Autodesk Inventor part; units mm, degrees
ref_plane "YZ Plane" through (0, 0, 0) normal (1, 0, 0) x (0, 1, 0)
ref_plane "XZ Plane" through (0, 0, 0) normal (0, 1, 0) x (-1, 0, 0)
ref_plane "XY Plane" through (0, 0, 0) normal (0, 0, 1) x (1, 0, 0)
ref_plane "Work Plane1" through (0, 0, 0) normal (0, 0, 1) x (1, 0, 0)
sketch "Sketch1" plane through (0, 0, 0) normal (0, 0, 1) x (1, 0, 0)
  circle A0 centre (0, 0) radius 25.9979
  circle A1 centre (-9.4998, -11.0022) radius 2.6601
  circle A2 centre (0.0001, -0.0022) radius 3.8801
  circle A3 centre (0.0001, -0.0022) radius 6.7754
  point P0 (0, 0)
extrude "Extrusion1" add sketch "Sketch1" along normal blind 7 contours A0
sketch "Sketch2" plane through (0, 0, 7) normal (0, 0, 1) x (1, 0, 0)
  line L0 (-10.4551, 50.2837) -> (48.898, -9.0695)
  line L1 (48.898, -9.0695) -> (20.6137, -37.3537)
  line L2 (20.6137, -37.3537) -> (-38.7394, 21.9994)
  line L3 (-38.7394, 21.9994) -> (-10.4551, 50.2837)
  line L4 (-10.4551, 50.2837) -> (20.6137, -37.3537) construction
  line L5 (48.898, -9.0695) -> (-38.7394, 21.9994) construction
  line L6 (-10.4551, 50.2837) -> (73.4829, 50.2837) construction
  circle A0 centre (-9.4998, -11.0022) radius 2.6601
  point P0 (5.0793, 6.465)
  dimension "d2" = 135
  dimension "d3" = 40
extrude "Extrusion2" cut sketch "Sketch2" against normal blind 2.5 contours L0 L1 L2 L3
sketch "Sketch3" plane through (0, 0, 7) normal (0, 0, 1) x (1, 0, 0)
  line L0 (-7.7936, -20.2561) -> (-2.9652, -15.4277)
  line L1 (-18.7537, -9.2959) -> (-13.9253, -4.4675)
  line L2 (-13.219, -3.6198) -> (-2.1175, -14.7214)
  line L3 (-2.1175, -14.7214) -> (-8.2078, -20.8117)
  line L4 (-8.2078, -20.8117) -> (-19.3094, -9.7102)
  line L5 (-19.3094, -9.7102) -> (-13.219, -3.6198)
  line L6 (-7.6188, -9.1212) -> (-24.7373, 7.9973)
  line L7 (-13.1696, -3.5704) -> (-2.1175, -14.7214)
  line L8 (-2.1175, -14.7214) -> (-0.0463, -12.6686)
  line L9 (-0.0463, -12.6686) -> (-11.0984, -1.5176)
  line L10 (-11.0984, -1.5176) -> (-13.1696, -3.5704)
  line L11 (-13.1696, -3.5704) -> (-13.219, -3.6198)
  line L12 (7.9973, -24.7373) -> (-24.7373, 7.9973)
  line L13 (-13.9253, -4.4675) -> (-2.9652, -15.4277)
  line L14 (-7.7936, -20.2561) -> (-18.7537, -9.2959)
  point P0 (0, 0)
  point P1 (-8.9176, -8.4066)
  point P2 (-24.7373, 7.9973)
  dimension "d6" = 0.1
extrude "Extrusion3" cut sketch "Sketch3" against normal up to surface (2.5 mm away) contours L14 L1 L13 L0 | L11 L7 L2 | L2 L3 L4 L5 | L7 L6 L12 L8 | L10 L9 L8 L12 L6
sketch "Skizze4" plane through (0, 0, 7) normal (0, 0, 1) x (1, 0, 0)
  spline S0 degree 2 poles (24.1427, 2.2394) (24.731, 1.8489) (25.3785, 0.5587) (25.3785, -0.3311) knots 0 0 0 1 2 2 2 construction
  spline S1 degree 2 poles (25.3785, -0.3311) (25.3785, -1.1665) (24.7013, -2.5111) (24.1328, -2.8867) knots 0 0 0 1 2 2 2 construction
  spline S2 degree 2 poles (24.1328, -2.8867) (23.6682, -3.1784) (22.7141, -3.3761) (21.9726, -3.3761) knots 0 0 0 1 2 2 2 construction
  line L0 (21.9726, -3.3761) -> (20.5687, -3.3761) construction
  line L1 (20.5687, -3.3761) -> (20.5687, 2.7239) construction
  line L2 (20.5687, 2.7239) -> (21.9578, 2.7239) construction
  spline S3 degree 2 poles (21.9578, 2.7239) (22.8179, 2.7239) (23.7967, 2.4668) (24.1427, 2.2394) knots 0 0 0 1 2 2 2 construction
  spline S4 degree 2 poles (19.1896, -2.9312) (18.8979, -3.1982) (18.1564, -3.4849) (17.5978, -3.4849) knots 0 0 0 1 2 2 2 construction
  spline S5 degree 2 poles (17.5978, -3.4849) (16.9354, -3.4849) (16.0061, -3.2081) (15.5958, -3.0103) knots 0 0 0 1 2 2 2 construction
  line L3 (15.5958, -3.0103) -> (15.5958, -1.992) construction
  line L4 (15.5958, -1.992) -> (15.6551, -1.992) construction
  spline S6 degree 2 poles (15.6551, -1.992) (16.0555, -2.3677) (17.0689, -2.7829) (17.5385, -2.7829) knots 0 0 0 1 2 2 2 construction
  spline S7 degree 2 poles (17.5385, -2.7829) (18.2108, -2.7829) (18.8979, -2.2243) (18.8979, -1.7646) knots 0 0 0 1 2 2 2 construction
  spline S8 degree 2 poles (18.8979, -1.7646) (18.8979, -1.3988) (18.5371, -0.944) (18.1465, -0.8303) knots 0 0 0 1 2 2 2 construction
  spline S9 degree 2 poles (18.1465, -0.8303) (17.8648, -0.7513) (17.3952, -0.6425) (17.0442, -0.5535) knots 0 0 0 1 2 2 2 construction
  spline S10 degree 2 poles (17.0442, -0.5535) (16.7278, -0.4695) (16.2285, -0.2174) (16.0358, -0.0147) knots 0 0 0 1 2 2 2 construction
  spline S11 degree 2 poles (16.0358, -0.0147) (15.8479, 0.188) (15.6403, 0.7317) (15.6403, 1.0876) knots 0 0 0 1 2 2 2 construction
  spline S12 degree 2 poles (15.6403, 1.0876) (15.6403, 1.8291) (16.797, 2.8326) (17.6918, 2.8326) knots 0 0 0 1 2 2 2 construction
  spline S13 degree 2 poles (17.6918, 2.8326) (18.2059, 2.8326) (19.1154, 2.6299) (19.5059, 2.4372) knots 0 0 0 1 2 2 2 construction
  line L5 (19.5059, 2.4372) -> (19.5059, 1.4683) construction
  line L6 (19.5059, 1.4683) -> (19.4466, 1.4683) construction
  spline S14 degree 2 poles (19.4466, 1.4683) (19.155, 1.7352) (18.2454, 2.1307) (17.7461, 2.1307) knots 0 0 0 1 2 2 2 construction
  spline S15 degree 2 poles (17.7461, 2.1307) (17.1826, 2.1307) (16.4856, 1.6017) (16.4856, 1.1717) knots 0 0 0 1 2 2 2 construction
  spline S16 degree 2 poles (16.4856, 1.1717) (16.4856, 0.7861) (16.8959, 0.3264) (17.2815, 0.2226) knots 0 0 0 1 2 2 2 construction
  spline S17 degree 2 poles (17.2815, 0.2226) (17.5385, 0.1534) (18.285, -0.0246) (18.5321, -0.0987) knots 0 0 0 1 2 2 2 construction
  spline S18 degree 2 poles (18.5321, -0.0987) (19.1599, -0.2915) (19.7432, -1.0676) (19.7432, -1.6361) knots 0 0 0 1 2 2 2 construction
  spline S19 degree 2 poles (19.7432, -1.6361) (19.7432, -1.997) (19.4516, -2.689) (19.1896, -2.9312) knots 0 0 0 1 2 2 2 construction
  circle A0 centre (-9.9998, 17.4978) radius 1.3999 construction
  circle A1 centre (10.0001, 17.4979) radius 1.4 construction
  circle A2 centre (10.0001, -17.5021) radius 1.4 construction
  circle A3 centre (-9.9998, -17.5021) radius 1.4001 construction
  arc A4 (-25.1198, 6.6998) -> (-24.1417, 5.4917) centre (-24.1417, 6.4917) ccw construction
  line L7 (-24.1417, 5.4917) -> (-17.7002, 5.4917) construction
  arc A5 (-15.7002, 3.4917) -> (-17.7002, 5.4917) centre (-17.7002, 3.4917) ccw construction
  line L8 (-15.7002, 3.4917) -> (-15.7002, -4.496) construction
  arc A6 (-17.7002, -6.496) -> (-15.7002, -4.496) centre (-17.7002, -4.496) ccw construction
  line L9 (-17.7002, -6.496) -> (-23.8502, -6.496) construction
  arc A7 (-23.8502, -6.496) -> (-24.8235, -7.7254) centre (-23.8502, -7.496) ccw construction
  arc A8 (-24.8235, -7.7254) -> (-25.1198, 6.6998) centre (0, 0) ccw construction
  circle A9 centre (-9.4998, -11.0022) radius 2.6601 construction
  circle A10 centre (-16.8291, -16.0482) radius 1.4 construction
  circle A11 centre (6.1284, 23.0202) radius 1.4 construction
  circle A12 centre (22.7119, 7.1872) radius 1.4 construction
  circle A13 centre (0.0001, -0.0022) radius 6.5 construction
  point P0 (0, 0)
hole "Bohrung1" at (6.1284, 23.0202, 7) at (22.7119, 7.1872, 7) at (-16.8291, -16.0482, 7) direction (0, 0, -1) diameter 3.2 end through all counterbore diameter 6.5 counterbore depth 5.5
sketch "Skizze5" plane through (0, 0, 4.5) normal (0, 0, 1) x (1, 0, 0)
  circle A0 centre (0.0001, -0.0022) radius 6.7754
  circle A1 centre (3.9139, 5.5285) radius 18
  point P0 (0, 0)
  dimension "d16" = 36
properties part number "Matchboxscope_sample_universal"
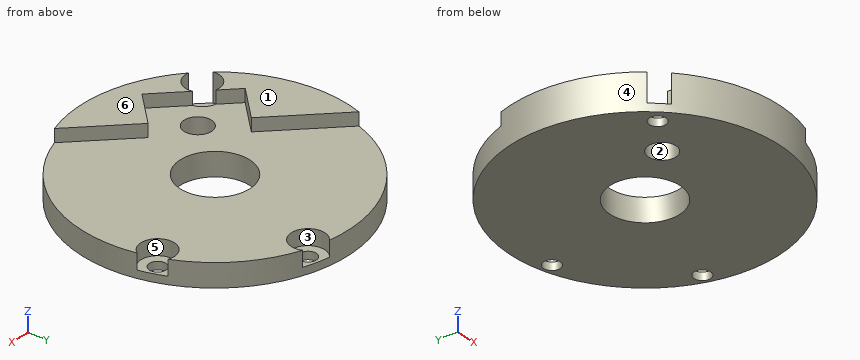
Part model, mm, in its own coordinate system. Face numbers are marked on the shaded views. A direction names the side the tool comes from. Round coordinates to 2 decimals unless told otherwise and drop trailing zeros. Write each loop counter-clockwise with the first axis right and the second up, starting at its lowest first coordinate (ties: lowest second). Pieces come first, ordered by that corner, then holes. Notation, with made-up numbers: (0.5, 81) -> (37.5, 81) arc R23 ccw to (37.5, 90) -> close; hole circle Ø9 at (-32, 43). An arc over 180 degrees is marked (long way). Return JSON: item names as keys, results as strings. Group by question number.
Q1. Mould opens along X. For the marked faces 1, 2, 3 and 4 say: pulls with the +X half, pulls with the -X half, needs draft (parallel to the pull), parting line crosses it, or undercut.
Q2. Saw through at D-D on x = 17. Write the cut outline in (y, z), plus the area to 3 significant figures.
Q3. Saw through at C-C on z = 0.75. Write the cut outline in (x, y).
Q4. Probe L1, parallel to Y at x = -17, z = 6.75; L2, parallel to Z at x = 9, y = 15; L3, parallel to X at y = -2, z = 0.5. List the from-to ranges inside material, lowest first. Write a range as [from, to].
Q5. Saw through at B-B on z = 5.5. Write the cut outline in (x, y), plus the area to 3 significant figures.
Q6. Pin check, flat tips, straight feed: pin 1 (8 mm diameter, centred on x = 0, y = -4.5, fed in from +Z); pin 2 (4 mm diameter, centred on x = -17.5, z = 3, fed in from +Y); pin 3 (3 mm diameter, centred on x = -15, z = 5, fed in from +Y). Stop position of each tip, or through.
Q7. Which spindle directions (+Z, -Z, +X, -X, +Y, -Y) get a long thin tool onto all of the face, cutting with end or side? Do the marked faces 5 and 6. Say none if no direction does.
Q8. Saw through at A-A on x = 0. Write the cut outline in (y, z), plus the area to 3 significant figures.
Answer:
{
 "1": {"face 1": "needs draft", "face 2": "undercut", "face 3": "undercut", "face 4": "parting line crosses it"},
 "2": {"outline": "(-19.67, 0) -> (19.67, 0) -> (19.67, 4.5) -> (-19.67, 4.5) -> close", "area": "177 mm2"},
 "3": {"outline": "circle Ø52 at (0, 0); hole circle Ø3.2 at (-16.83, -16.05); hole circle Ø5.32 at (-9.5, -11); hole circle Ø13.55 at (0, 0); hole circle Ø3.2 at (6.13, 23.02); hole circle Ø3.2 at (22.71, 7.19)"},
 "4": {"L1": "[-19.67, -19.29], [-12.8, -12.02], [-7.4, 0.26]", "L2": "[0, 4.5]", "L3": "[-25.92, -6.47], [6.47, 25.92]"},
 "5": {"outline": "(-24.74, 8) arc R26 ccw to (-20.04, -16.56) arc R3.25 cw to (-16.15, -12.87) -> (-19.31, -9.71) -> (-13.17, -3.57) -> close; (-17.5, -19.23) arc R26 ccw to (8, -24.74) -> (-2.07, -14.67) -> (-2.12, -14.72) -> (-8.21, -20.81) -> (-13.65, -15.37) arc R3.25 cw to start", "area": "301 mm2"},
 "6": {"pin 1": "z = 4.5", "pin 2": "y = 20.87", "pin 3": "y = 22.17"},
 "7": {"face 5": "+Z", "face 6": "+Z, +X, -X, +Y, -Y"},
 "8": {"outline": "(-26, 0) -> (-6.78, 0) -> (-6.78, 4.5) -> (-16.74, 4.5) -> (-16.74, 7) -> (-26, 7) -> close; (6.77, 0) -> (26, 0) -> (26, 4.5) -> (6.77, 4.5) -> close", "area": "196 mm2"}
}
